Input: part model. Units: mm. Frame: model coordinates. Face numbers are marked on the shaded views. Round coordinates to 2 decimals unless told otherwise and drop trailing zeros. Write each loop counter-clockwise with the first axis right and the second up, starting at its lowest first coordinate (ties: lowest second). Pieces come first, ordered by that corner, then holes. Notation, with made-up numbers: (5.25, 44.25) -> (21.25, 44.25) arc R17 ccw to (21.25, 71.25) -> close; hole circle Ø5 at (76.5, 31). An arc over 180 degrees is marked (long way). Write item = value, one per line.
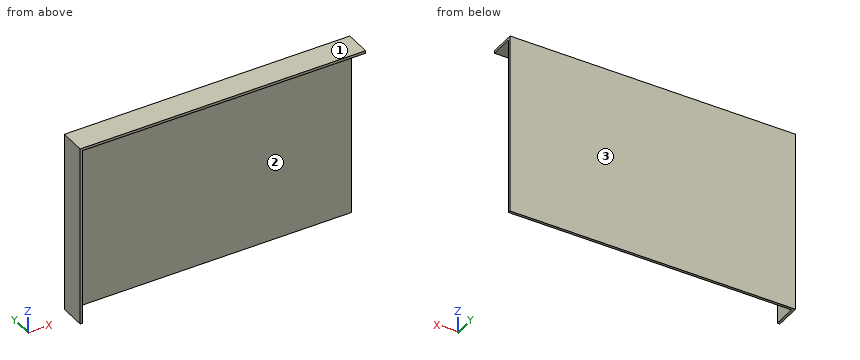
```python
from build123d import *

# Parameters (mm, degrees)
BOSS_EXTRUDE1_DEPTH = 25.4
FILLET1_R           = 20.32
SHELL1_T            = -2.54
SKETCH2_R           = 2.54
CUT_EXTRUDE1_DEPTH  = 347.409815103
SKETCH3_R           = 2.54
CUT_EXTRUDE2_DEPTH  = 347.409815103


with BuildPart() as part:
    # Sketch1 → Boss-Extrude1 (new body)
    with BuildSketch(Plane(origin=(0, 0, 0), x_dir=(1, 0, 0), z_dir=(0, 1, 0))):
        Polygon((-279.4, 203.2), (-279.4, -203.2), (279.4, -203.2), (279.4, 203.2), (152.4, 203.2), (152.4, 12.7), (-152.4, 12.7), (-152.4, 203.2), align=None)
    extrude(amount=BOSS_EXTRUDE1_DEPTH)

    # Fillet1
    fillet1_edges = [part.edges().sort_by_distance(p)[0] for p in [
        (279.4, 12.7, -203.2),
        (-279.4, 12.7, -203.2),
        (-152.4, 12.7, -203.2),
        (152.4, 12.7, -203.2),
    ]]
    fillet(fillet1_edges, radius=FILLET1_R)

    # Shell1
    shell1_openings = [part.faces().sort_by_distance(p)[0] for p in [
        (0, 0, 37.577423361),
    ]]
    offset(amount=SHELL1_T, openings=shell1_openings, kind=Kind.INTERSECTION)

    # Sketch2 → Cut-Extrude1 (cut, through all)
    with BuildSketch(Plane(origin=(0, 25.4, 0), x_dir=(1, 0, 0), z_dir=(0, 1, 0))):
        with Locations(Location((-177.72, 165.1, 0), (0, 0, 270))):
            Circle(SKETCH2_R)
        with Locations(Location((-167.56, 165.1, 0), (0, 0, 270))):
            Circle(SKETCH2_R)
        with Locations(Location((167.56, 165.1, 0), (0, 0, 270))):
            Circle(SKETCH2_R)
        with Locations(Location((177.72, 165.1, 0), (0, 0, 270))):
            Circle(SKETCH2_R)
    extrude(amount=-CUT_EXTRUDE1_DEPTH, mode=Mode.SUBTRACT)

    # Sketch3 → Cut-Extrude2 (cut, through all)
    with BuildSketch(Plane(origin=(0, 25.4, 0), x_dir=(1, 0, 0), z_dir=(0, 1, 0))):
        with BuildLine():
            Line((-279.4, 182.88), (-279.4, -25.4))
            Line((-279.4, -25.4), (0, -25.4))
            Line((0, -25.4), (0, -203.2))
            Line((0, -203.2), (279.4, -203.2))
            Line((279.4, -203.2), (279.4, 182.88))
            ThreePointArc((279.4, 182.88), (273.448409794, 197.248409794), (259.08, 203.2))
            Line((259.08, 203.2), (172.72, 203.2))
            ThreePointArc((172.72, 203.2), (158.351590206, 197.248409794), (152.4, 182.88))
            Line((152.4, 182.88), (152.4, 12.7))
            Line((152.4, 12.7), (-152.4, 12.7))
            Line((-152.4, 12.7), (-152.4, 182.88))
            ThreePointArc((-152.4, 182.88), (-158.351590206, 197.248409794), (-172.72, 203.2))
            Line((-172.72, 203.2), (-259.08, 203.2))
            ThreePointArc((-259.08, 203.2), (-273.448409794, 197.248409794), (-279.4, 182.88))
        make_face()
        with Locations((-177.72, 165.1)):
            Circle(SKETCH3_R, mode=Mode.SUBTRACT)
        with Locations((-167.56, 165.1)):
            Circle(SKETCH3_R, mode=Mode.SUBTRACT)
        with Locations((167.56, 165.1)):
            Circle(SKETCH3_R, mode=Mode.SUBTRACT)
        with Locations((177.72, 165.1)):
            Circle(SKETCH3_R, mode=Mode.SUBTRACT)
    extrude(amount=-CUT_EXTRUDE2_DEPTH, mode=Mode.SUBTRACT)


solid = part.part
```
1) First-contact query: P1, Ø11.5, axis at y = 9.5, z = 96, coming from the +X side; P2, Ø1, axis at x = -52.5, y = 9.5, coming from the -Z side; P3, Ø12, axis at x = -90.5, z = 144.5, coming from the -Y side. Flat tips, straight axial feed; report the tip coordinate or a pass-through.
Solutions:
P1 = -276.86
P2 = 200.66
P3 = 22.86
2) Draft query along Y for the marked faces 1, 2 and 3. Return one class per face: +Y half, -Y half, draft (parallel to the pull), parting line (faces both ways), or undercut.
Solutions:
face_1 = draft
face_2 = -Y half
face_3 = +Y half
3) Cut plane B-B (x = -67). Return the cut outline in (y, z), and give its area (3 significant figures).
Solutions:
outline = (0, 200.66) -> (22.86, 200.66) -> (22.86, 25.4) -> (25.4, 25.4) -> (25.4, 203.2) -> (0, 203.2) -> close
area = 510 mm^2
4) Line query: L1, parallel to Z at x = -11.5, y = 21.5; L2, parallel to Y at x = -197, z = 163.5; L3, parallel to X at y = 10, z = 132. Output: solid intervals per line, ascending. Write a range as from..to.
Solutions:
L1 = 200.66..203.2
L2 = 22.86..25.4
L3 = -279.4..-276.86
5) Cut plane A-A (z = 147). Return the cut outline in (x, y), and give its area (3 significant figures).
Solutions:
outline = (-279.4, 0) -> (-276.86, 0) -> (-276.86, 22.86) -> (0, 22.86) -> (0, 25.4) -> (-279.4, 25.4) -> close
area = 768 mm^2
